```python
from build123d import *

# Parameters (mm, degrees)
CROQUIS1_W              = 203
CROQUIS1_H              = 205
SALIENTE_EXTRUIR1_DEPTH = 173
CROQUIS2_W              = 172
CROQUIS2_H              = 140
CORTAR_EXTRUIR1_DEPTH   = 211
CORTAR_EXTRUIR2_DEPTH   = 33
VACIADO1_START          = 5
VACIADO1_DEPTH          = 163
CROQUIS6_R              = 27
CORTAR_EXTRUIR4_DEPTH   = 5
CROQUIS8_R              = 6
CORTAR_EXTRUIR5_DEPTH   = 5


# Read off the part's stored shape, not the designer's step: Vaciado1
with BuildPart() as part:
    # Croquis1 → Saliente-Extruir1 (new body)
    with BuildSketch(Plane(origin=(0, 0, 0), x_dir=(1, 0, 0), z_dir=(0, 1, 0))):
        with Locations((0, 19.601485149)):
            Rectangle(CROQUIS1_W, CROQUIS1_H)
    extrude(amount=SALIENTE_EXTRUIR1_DEPTH)

    # Croquis2 → Cortar-Extruir1 (cut)
    with BuildSketch(Plane.ZY.offset(101.5)):
        with Locations((-3.101485149, 103)):
            Rectangle(CROQUIS2_W, CROQUIS2_H)
    extrude(amount=-CORTAR_EXTRUIR1_DEPTH, mode=Mode.SUBTRACT)

    # Croquis3 → Cortar-Extruir2 (cut)
    with BuildSketch(Plane(origin=(0, 33, 0), x_dir=(1, 0, 0), z_dir=(0, 1, 0))):
        with BuildLine():
            Line((-101.5, 3.101485149), (-101.5, -82.898514851))
            Line((-101.5, -82.898514851), (-88.5, -82.898514851))
            Line((-88.5, -82.898514851), (-4.929378531, -82.898514851))
            ThreePointArc((-4.929378531, -82.898514851), (-64.166087143, -56.856935388), (-88.5, 3.101485149))
            Line((-88.5, 3.101485149), (-101.5, 3.101485149))
        make_face()
        with BuildLine():
            ThreePointArc((88.5, 3.101485149), (60.988030108, -57.123115602), (0, -82.898514851))
            Line((0, -82.898514851), (88.5, -82.898514851))
            Line((88.5, -82.898514851), (101.5, -82.898514851))
            Line((101.5, -82.898514851), (101.5, 3.101485149))
            Line((101.5, 3.101485149), (88.5, 3.101485149))
        make_face()
    extrude(amount=-CORTAR_EXTRUIR2_DEPTH, mode=Mode.SUBTRACT)

    # Vaciado1 outline → Vaciado1 (cut)
    with BuildSketch(Plane(origin=(0, 0, 0), x_dir=(1, 0, 0), z_dir=(0, 1, 0)).offset(VACIADO1_START)):
        with BuildLine():
            Line((-96.5, 8.101485149), (-83.345599163, 8.101485149))
            ThreePointArc((-83.345599163, 8.101485149), (-62.319461008, -51.525686528), (-4.856672926, -77.898514851))
            Line((-4.856672926, -77.898514851), (-0.072642407, -77.898514851))
            ThreePointArc((-0.072642407, -77.898514851), (59.19666813, -51.84566757), (83.649498309, 8.101485149))
            Line((83.649498309, 8.101485149), (96.5, 8.101485149))
            Line((96.5, 8.101485149), (96.5, 117.101485149))
            Line((96.5, 117.101485149), (-96.5, 117.101485149))
            Line((-96.5, 117.101485149), (-96.5, 8.101485149))
        make_face()
    extrude(amount=VACIADO1_DEPTH, mode=Mode.SUBTRACT)

    # Croquis6 → Cortar-Extruir4 (cut)
    with BuildSketch(Plane(origin=(0, 0, -122.101485149), x_dir=(-1, 0, 0), z_dir=(0, 0, -1))):
        with Locations((-31.5, 48)):
            Circle(CROQUIS6_R)
    extrude(amount=-CORTAR_EXTRUIR4_DEPTH, mode=Mode.SUBTRACT)

    # Croquis8 → Cortar-Extruir5 (cut)
    with BuildSketch(Plane.XZ):
        with Locations(Location((-31.5, -70.101485149, 0), (0, 0, 270))):
            Circle(CROQUIS8_R)
        with Locations(Location((-31.5, -18.101485149, 0), (0, 0, 270))):
            Circle(CROQUIS8_R)
        with Locations(Location((-31.5, 33.898514851, 0), (0, 0, 270))):
            Circle(CROQUIS8_R)
        with Locations(Location((31.5, -18.101485149, 0), (0, 0, 270))):
            Circle(CROQUIS8_R)
        with Locations(Location((31.5, 33.898514851, 0), (0, 0, 270))):
            Circle(CROQUIS8_R)
        with Locations(Location((31.5, -70.101485149, 0), (0, 0, 270))):
            Circle(CROQUIS8_R)
    extrude(amount=-CORTAR_EXTRUIR5_DEPTH, mode=Mode.SUBTRACT)


solid = part.part
```
Source: CAD feature listing. Evaluate the final solid. Frame: model axes, mm. A direction names the side the tool comes from. Coordinates: 2 decimals unless noted, no trailing zeros. Loops run counter-clockwise (first coordinate to the right, second up) from the corner with the lowest first, then second, coordinate; pieces in that order, holes last. Notation, with made-up numbers: M -39,-31 L -9,-31 A27 cw -9,1 Z; hole C 74,-19 d7. An arc over 180 degrees is marked long. Put each result on its own line as item: value. Start each with the question number.
1) Cut plane D-D on x = 31.5. Return the cut outline in (y, z).
2) Cut plane A-A on y = 48. Return the cut outline in (x, z), then the cut area to 4 significant figures.
3) Ray query, L1, parallel to Y at x = -46, z = -21; L2, parallel to Y at x = -9.5, z = -92; L3, parallel to Z at x = -20.5, y = 143. Return the intervals inside material, ascending. Write a range as from..to.
4) Reachability of faces 1 (the face through (58.545, 18.804, 52.508)), 2 (the face through (-1, 168, -103)), 3 (the face through (96.5, 49, -98)) from +Z, -Z, +X, -X, +Y, -Y: full face, straight path, thin tool, end or side. Return the list, or none.
5) Cut plane B-B on z = -109. Return the cut outline in (x, y), then the cut area to 3 significant figures.
6) Contact query for flat-ended pins moving along their axis: pin 1 Ø19 at (x, z) = (-31.5, 33.9) entering from +Y; pin 2 Ø4 at (x, y) = (76.5, 118) entering from +Z; pin 3 Ø3 at (y, z) = (20.5, 12) entering from -X. Output: stop coordinate, or through.
7) Pull-direction query (Y, two-part tool) for faces 4 (the face through (-1, 5, -21)), 5 (the face through (-96.5, 49, -100)), 6 (the face through (31.764, 2.465, -64.107)), 7 (the face through (-1, 173, -106)); classes: pulls with the +Y half, pulls with the -Y half, needs draft (parallel to the pull), parting line crosses it, or undercut.
8) Cut plane C-C on x = 8.5. Return the cut outline in (y, z), then the cut area to 3 significant figures.
The answers:
1. outline: M 0,-122.1 L 21,-122.1 L 21,-117.1 L 5,-117.1 L 5,-76.1 L 0,-76.1 Z; M 0,-64.1 L 5,-64.1 L 5,-24.1 L 0,-24.1 Z; M 0,-12.1 L 5,-12.1 L 5,27.9 L 0,27.9 Z; M 0,39.9 L 5,39.9 L 5,70.9 L 33,70.9 L 33,76.32 L 0,76.32 Z; M 75,-122.1 L 173,-122.1 L 173,-89.1 L 168,-89.1 L 168,-117.1 L 75,-117.1 Z
2. outline: M -101.5,-122.1 L 4.5,-122.1 L 4.5,-117.1 L -96.5,-117.1 L -96.5,-89.1 L -101.5,-89.1 Z; M 58.5,-122.1 L 101.5,-122.1 L 101.5,-89.1 L 96.5,-89.1 L 96.5,-117.1 L 58.5,-117.1 Z
2. area: 1,025 mm²
3. L1: y = 0..5
3. L2: y = 0..5, 168..173
3. L3: z = -122.1..-117.1
4. face 1: +Y
4. face 2: +Z
4. face 3: none
5. outline: M -101.5,0 L 101.5,0 L 101.5,173 L -101.5,173 Z; hole M -96.5,5 L 96.5,5 L 96.5,168 L -96.5,168 Z
5. area: 3,660 mm²
6. pin 1: stops at y = 5
6. pin 2: stops at z = -117.1
6. pin 3: stops at x = -87.42
7. face 4: undercut
7. face 5: undercut
7. face 6: needs draft
7. face 7: pulls with the +Y half
8. outline: M 0,-122.1 L 33.86,-122.1 L 33.86,-117.1 L 5,-117.1 L 5,77.22 L 33,77.22 L 33,82.26 L 0,82.26 Z; M 62.14,-122.1 L 173,-122.1 L 173,-89.1 L 168,-89.1 L 168,-117.1 L 62.14,-117.1 Z
8. area: 2,000 mm²
